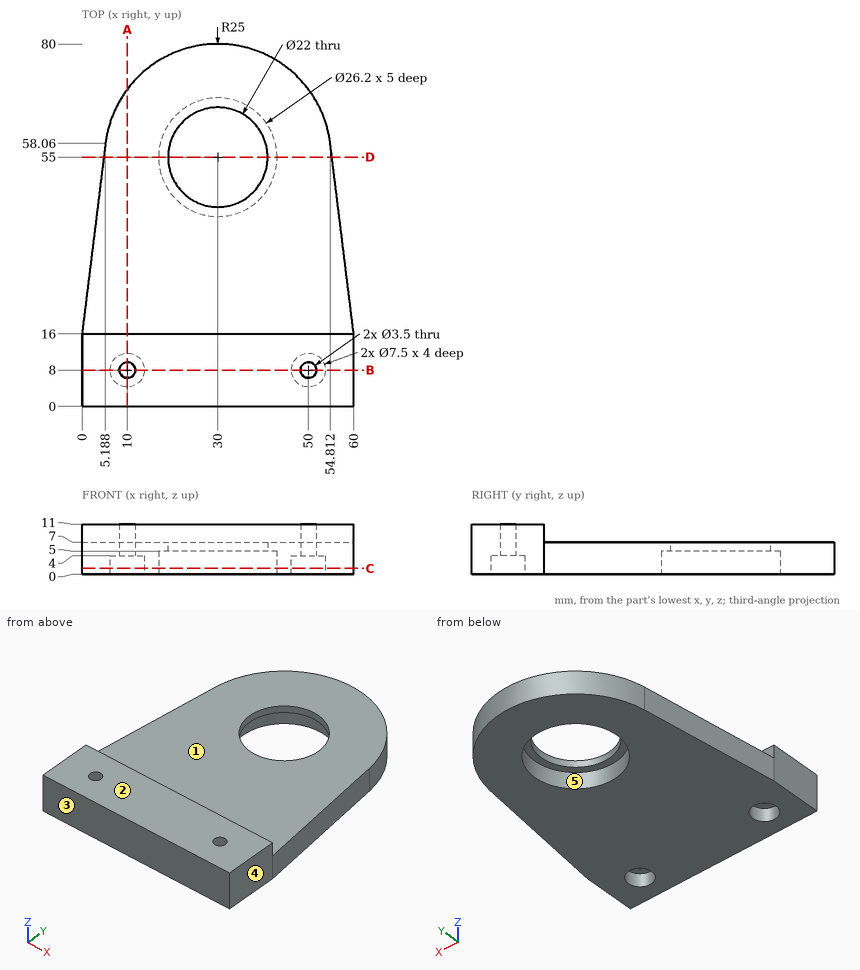
Geometry check sheet. Reference: drawing and pictorial views, mm from the part's lowest x, y, z. A direction names the side the tool comes from. Round coordinates to 2 decimals unless told otherwise and drop trailing zeros. Write each loop counter-clockwise with the first axis right and the second up, starting at its lowest first coordinate (ties: lowest second). Pieces come first, ordered by that corner, then holes. Notation, with made-up numbers: (-27, 74.5) -> (5, 74.5) arc R9 ccw to (5, 82.5) -> close; hole circle Ø3 at (77.25, -2). An arc over 180 degrees is marked (long way). Put each result on its own line as item: value.
1) Cross-section at D-D, the plane y = 55. Enter the section's corners in (x, z), plus the area to 3 significant figures.
Recorded:
outline: (4.81, 0) -> (16.9, 0) -> (16.9, 5) -> (19, 5) -> (19, 7) -> (4.81, 7) -> close; (41, 5) -> (43.1, 5) -> (43.1, 0) -> (55.19, 0) -> (55.19, 7) -> (41, 7) -> close
area: 178 mm2
2) Depth check by flat-ended pin: P1, Ø3, axis at x = 30, z = 9.5, coming from the +Y side; P2, Ø6, axis at x = 12, y = 47, coming from the +Z side; P3, Ø4, axis at x = 50, y = 8, coming from the -Z side. Enter the tip coordinate at first touch or a pass-through.
Recorded:
P1: stops at y = 16
P2: stops at z = 7
P3: stops at z = 4
3) Cross-section at B-B, the plane y = 8. Enter the section's corners in (x, z), plus the area to 3 significant figures.
Recorded:
outline: (0, 0) -> (6.25, 0) -> (6.25, 4) -> (8.25, 4) -> (8.25, 11) -> (0, 11) -> close; (11.75, 4) -> (13.75, 4) -> (13.75, 0) -> (46.25, 0) -> (46.25, 4) -> (48.25, 4) -> (48.25, 11) -> (11.75, 11) -> close; (51.75, 4) -> (53.75, 4) -> (53.75, 0) -> (60, 0) -> (60, 11) -> (51.75, 11) -> close
area: 551 mm2
4) Release check for a two-part mould opening along X. For the marked faces 3, 4 and 5 record: pulls with the +X half, pulls with the -X half, needs draft (parallel to the pull), parting line crosses it, or undercut.
Recorded:
face 3: needs draft
face 4: pulls with the +X half
face 5: undercut
5) Access from +Z, -Z, +X, -X, +Y, -Y to the whole of each face (thin tool, end or side, straight path). Record for the marked faces 1 and 2.
Recorded:
face 1: +Z, +X, -X, +Y
face 2: +Z, +X, -X, +Y, -Y
6) Cross-section at A-A, the plane x = 10. Enter the section's corners in (y, z).
Recorded:
outline: (0, 0) -> (4.25, 0) -> (4.25, 4) -> (6.25, 4) -> (6.25, 11) -> (0, 11) -> close; (9.75, 4) -> (11.75, 4) -> (11.75, 0) -> (70, 0) -> (70, 7) -> (16, 7) -> (16, 11) -> (9.75, 11) -> close
7) Cross-section at C-C, the plane z = 1.25. Enter the section's corners in (x, y), plus the area to 3 significant figures.
Recorded:
outline: (0, 0) -> (60, 0) -> (60, 16) -> (54.81, 58.06) arc R25 ccw to (5.19, 58.06) -> (0, 16) -> close; hole circle Ø7.5 at (10, 8); hole circle Ø26.2 at (30, 55); hole circle Ø7.5 at (50, 8)
area: 3,470 mm2
8) Thickness scan on probe 1 along X at (y, z) = (8, 9.25); probe 2 along Y at (x, z) = (30, 6.2); probe 3 along Y at (x, z) = (32.5, 7.75). Record the ranges inside material, lowest first. Write a range as from..to.
Recorded:
probe 1: x = 0..8.25, 11.75..48.25, 51.75..60
probe 2: y = 0..44, 66..80
probe 3: y = 0..16
